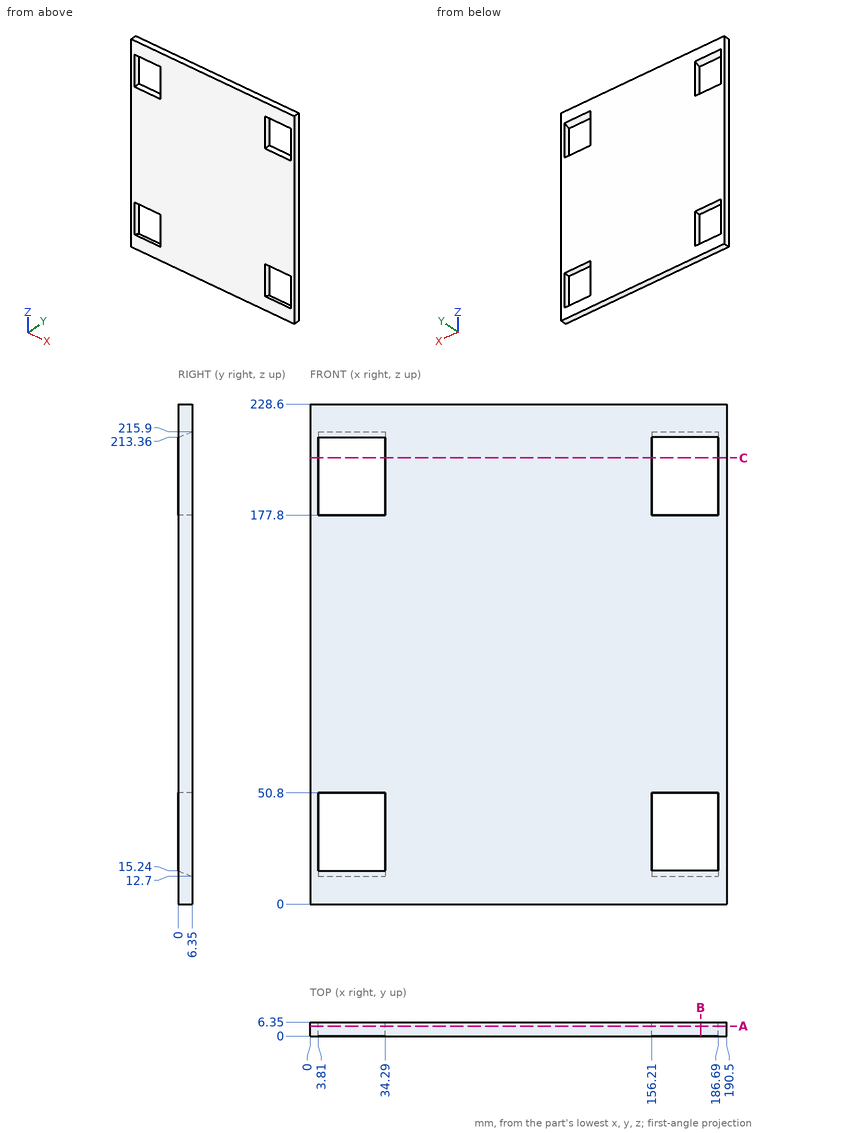
The drawing under review shows one solid part. Ordinate dimensions are in mm from its lowest x, y, z. Round coordinates to 2 decimals unless told otherwise and drop trailing zeros. Loops run counter-clockwise (first coordinate to the right, second up) from the corner with the lowest first, then second, coordinate; pieces in that order, holes last. Notation, with made-up numbers: (-36.75, -38) - (3.25, -38) arc R37 ccw to (3.25, -1) - close; hole circle Ø4 at (63, 2). An arc over 180 degrees is marked (long way). Use one line per item in the form item = value.
Item 1: Consider section C-C on z = 204. Write out the cut boundary in (x, y), then the cut area to 3 significant figures.
Answers:
outline = (0, 0) - (3.81, 0) - (3.81, 6.35) - (0, 6.35) - close; (34.29, 0) - (156.21, 0) - (156.21, 6.35) - (34.29, 6.35) - close; (186.69, 0) - (190.5, 0) - (190.5, 6.35) - (186.69, 6.35) - close
area = 823 mm^2
Item 2: Consider section B-B on x = 178.5. Write out the cut boundary in (y, z).
Answers:
outline = (0, 0) - (6.35, 0) - (6.35, 12.7) - (0, 15.24) - close; (0, 50.8) - (6.35, 50.8) - (6.35, 177.8) - (0, 177.8) - close; (0, 213.36) - (6.35, 215.9) - (6.35, 228.6) - (0, 228.6) - close
Item 3: Consider section A-A on y = 4.5. Write out the cut boundary in (x, z).
Answers:
outline = (0, 0) - (190.5, 0) - (190.5, 228.6) - (0, 228.6) - close; hole (3.81, 13.44) - (34.29, 13.44) - (34.29, 50.8) - (3.81, 50.8) - close; hole (3.81, 177.8) - (34.29, 177.8) - (34.29, 215.16) - (3.81, 215.16) - close; hole (156.21, 13.44) - (186.69, 13.44) - (186.69, 50.8) - (156.21, 50.8) - close; hole (156.21, 177.8) - (186.69, 177.8) - (186.69, 215.16) - (156.21, 215.16) - close
Item 4: For line 1 (X direction, y = 5.75, z = 22.5); line 2 (Z direction, x = 23.5, y = 1.5); line 3 (Z direction, x = 12.5, y = 3), list the stretches that pass through material, from the lowest coordinate up.
Answers:
line_1 = 0 to 3.81, 34.29 to 156.21, 186.69 to 190.5
line_2 = 0 to 14.64, 50.8 to 177.8, 213.96 to 228.6
line_3 = 0 to 14.04, 50.8 to 177.8, 214.56 to 228.6
